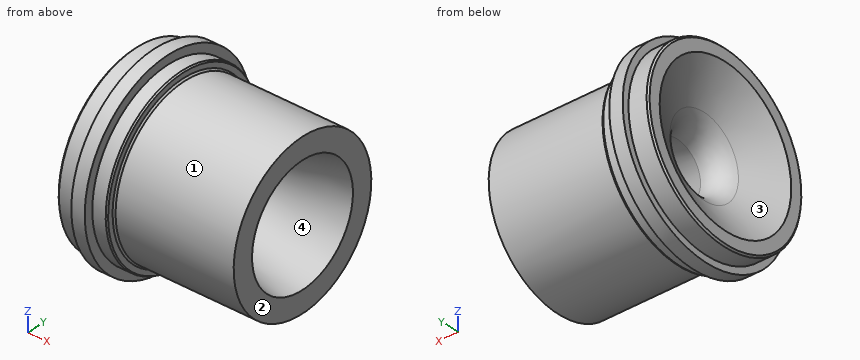
from build123d import *

# Parameters (mm, degrees)
CUT_EXTRUDE1_DEPTH      = 124.385507346
CUT_EXTRUDE1_DEPTH_BACK = 124.385507346
SKETCH2_W               = 25.452213303
SKETCH2_H               = 76.2


with BuildPart() as part:
    # Sketch1 → Revolve1 (revolve)
    with BuildSketch(Plane.XY, mode=Mode.PRIVATE) as revolve1_sk:
        with BuildLine():
            Line((0, 36.4109), (0, 41.9989))
            Line((0, 41.9989), (0.762, 42.7609))
            Line((0.762, 42.7609), (9.3472, 42.7609))
            Line((9.3472, 42.7609), (9.3472, 45.9613))
            Line((9.3472, 45.9613), (15.6972, 45.9613))
            Line((15.6972, 45.9613), (15.6972, 41.783))
            Line((15.6972, 41.783), (22.0472, 41.783))
            Line((22.0472, 41.783), (22.8092, 41.343059095))
            Line((22.8092, 41.343059095), (22.8092, 38.862))
            Line((22.8092, 38.862), (23.5712, 38.1))
            Line((23.5712, 38.1), (104.1146, 38.1))
            Line((104.1146, 38.1), (104.8766, 37.338))
            Line((104.8766, 37.338), (104.8766, 34.7599))
            Line((104.8766, 34.7599), (22.6314, 12.722365079))
            ThreePointArc((22.6314, 12.722365079), (15.406658957, 13.955510804), (10.066398525, 18.975386305))
            Line((10.066398525, 18.975386305), (0, 36.4109))
        make_face()
    revolve(revolve1_sk.sketch.rotate(Axis((0, 0, 0), (1, 0, 0)), 90), axis=Axis((0, 0, 0), (1, 0, 0)))

    # Sketch2 → Cut-Extrude1 (cut, two sides: drawn at the far end of the back side and taken through both)
    with BuildSketch(Plane.XY.offset(-CUT_EXTRUDE1_DEPTH_BACK)):
        with Locations((92.150493349, 0)):
            Rectangle(SKETCH2_W, SKETCH2_H)
    extrude(amount=CUT_EXTRUDE1_DEPTH + CUT_EXTRUDE1_DEPTH_BACK, mode=Mode.SUBTRACT)


solid = part.part
Verification items for the finished model (mm, model axes). Face numbers are marked on the shaded views. Give positions to 0.01 mm unless a question says otherwise; leave off trailing zeros. Loops run counter-clockwise (first coordinate to the right, second up) from the corner with the lowest first, then second, coordinate; pieces in that order, holes last. Notation, with made-up numbers: (-24.75, -28.75) - (-3.75, -28.75) arc R30 cw to (-3.75, 4.25) - close; hole circle Ø6 at (39.25, -16). An arc over 180 degrees is marked (long way). Write item = value, one per line. Start each with the question number.
Q1. Cross-section at D-D, the plane x = 67. Enter the section's corners in (y, z).
Q2. Mould release check, pull along Z, two halves, no side actions. Record for the marked faces 1, 2, 3 and 4: released by +Z, released by -Z, zero draft, split by the parting line, or undercut.
Q3. Depth check by flat-ended pin: P1, Ø4, axis at y = 24.5, z = -13, coming from the -X side; P2, Ø6, axis at y = -12.5, z = 2.5, coming from the -X side; P3, Ø4, axis at x = 46, z = 11, coming from the -Y side. Enter the tip coordinate at first touch or a pass-through.
Q4. Thickness scan on line 1 (Y direction, x = 24, z = -5); line 2 (X direction, y = 1.5, z = 40.5); line 3 (Z direction, x = 46, y = 3.5). Record the ranges inside material, lowest first.
Q5. Cross-section at C-C, the plane x = 38. Enter the section's corners in (y, z), and give its area (3 significant figures).
Answer key:
q1.outline = circle Ø76.2 at (0, 0); hole circle Ø49.22 at (0, 0)
q2.face_1 = split by the parting line
q2.face_2 = zero draft
q2.face_3 = undercut
q2.face_4 = undercut
q3.P1 = 3.85
q3.P2 = 12.72
q3.P3 = -37.02
q4.line_1 = -37.77 to -12.1, 12.1 to 37.77
q4.line_2 = 0 to 22.81
q4.line_3 = -37.94 to -18.66, 18.66 to 37.94
q5.outline = circle Ø76.2 at (0, 0); hole circle Ø33.68 at (0, 0)
q5.area = 3,670 mm^2
